The drawing under review shows one solid part. Ordinate dimensions are in mm from its lowest x, y, z. Coordinates: 2 decimals unless noted, no trailing zeros. Order: outer loops, then holes, each group sorted by start corner. A loop starts at its lowest first (then second) coordinate and runs counter-clockwise, first axis right, second up.
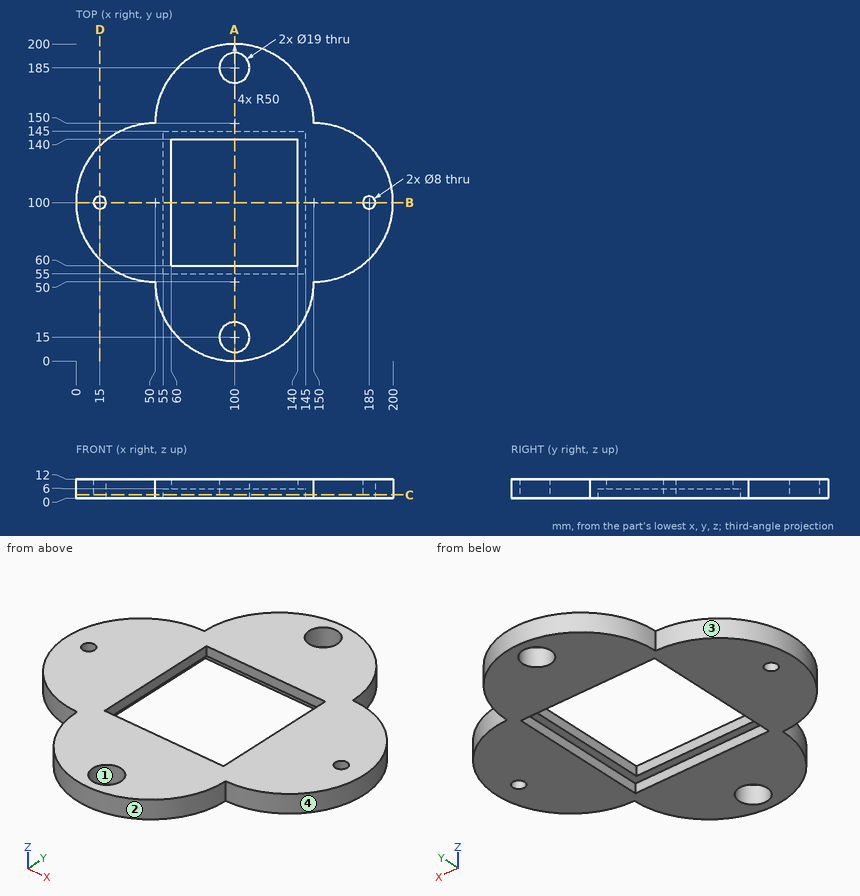
(1) The part is to be moulded in two halves that separate along X. For the marked faces 1, 2, 3 and 4, say which applies: +X half, -X half, draft (parallel to the pull), parting line (faces both ways), or undercut.
(2) Consider section D-D (x = 15). Give the boundary of the cut face in (y, z), then the cut area to 3 significant figures.
(3) Insertion check: pin 1 Ø5 at (y, z) = (89, 2.5) entering from +X; pin 2 Ø2 at (y, z) = (22.5, 8.5) entering from -X; pin 3 Ø5 at (y, z) = (105, 8) entering from +X; pin 4 Ø17 at (x, y) = (100, 185) entering from -Z. Each pin has a flat end and moves straight along its axis. Give the tip position at first contact, or say it passes through.
(4) Consider section B-B (y = 100). Give the boundary of the cut face in (x, z).
(5) Wall thickness on line 1 (Y direction, x = 100, z = 8); line 2 (Y direction, x = 96, z = 11); line 3 (X direction, y = 188, z = 7.25): over which ranges is each line inside the solid? List them lowest first.
(6) Consider section A-A (x = 100). Give the boundary of the cut face in (y, z).
(7) Consider section C-C (z = 2). Give the boundary of the cut face in (x, y), then the cut area to 3 significant figures.
Findings:
1. face 1: undercut
1. face 2: parting line
1. face 3: -X half
1. face 4: +X half
2. outline: (64.29, 0) - (96, 0) - (96, 12) - (64.29, 12) - close; (104, 0) - (135.71, 0) - (135.71, 12) - (104, 12) - close
2. area: 761 mm2
3. pin 1: stops at x = 199.27
3. pin 2: stops at x = 57.6
3. pin 3: stops at x = 199.94
3. pin 4: passes through
4. outline: (0, 0) - (11, 0) - (11, 12) - (0, 12) - close; (19, 0) - (55, 0) - (55, 6) - (60, 6) - (60, 12) - (19, 12) - close; (140, 6) - (145, 6) - (145, 0) - (181, 0) - (181, 12) - (140, 12) - close; (189, 0) - (200, 0) - (200, 12) - (189, 12) - close
5. line 1: y = 0 to 5.5, 24.5 to 60, 140 to 175.5, 194.5 to 200
5. line 2: y = 0.16 to 6.38, 23.62 to 60, 140 to 176.38, 193.62 to 199.84
5. line 3: x = 67.5 to 90.99, 109.01 to 132.5
6. outline: (0, 0) - (5.5, 0) - (5.5, 12) - (0, 12) - close; (24.5, 0) - (55, 0) - (55, 6) - (60, 6) - (60, 12) - (24.5, 12) - close; (140, 6) - (145, 6) - (145, 0) - (175.5, 0) - (175.5, 12) - (140, 12) - close; (194.5, 0) - (200, 0) - (200, 12) - (194.5, 12) - close
7. outline: (50, 50) arc R50 ccw to (150, 50) arc R50 ccw to (150, 150) arc R50 ccw to (50, 150) arc R50 ccw to start; hole circle Ø8 at (15, 100); hole (55, 55) - (145, 55) - (145, 145) - (55, 145) - close; hole circle Ø19 at (100, 15); hole circle Ø19 at (100, 185); hole circle Ø8 at (185, 100)
7. area: 16,900 mm2
